Check sheet for the modelled part. Datum: model origin and axes. Units: mm. Face numbers are marked on the shaded views. A direction names the side the tool comes from. Round coordinates to 2 decimals unless told otherwise and drop trailing zeros. Order: outer loops, then holes, each group sorted by start corner. A loop starts at its lowest first (then second) coordinate and runs counter-clockwise, first axis right, second up.
(1) Mould release check, pull along X, two halves, no side actions. Record for the marked faces 4, 5, 6 and 7: released by +X, released by -X, zero draft, split by the parting line, or undercut.
(2) Sectioned sample at C-C, the plane y = 10.9. Enter the section's corners in (x, z), and give its area (3 significant figures).
(3) Thickness scan on probe 1 along X at (y, z) = (14.75, 13); probe 2 along X at (y, z) = (11, 13); probe 3 along X at (y, z) = (11.75, 13). Record the ranges inside material, lowest first.
(4) Sectioned sample at D-D, the plane z = 9.75. Enter the section's corners in (x, y).
(5) Depth check by flat-ended pin: pin 1 (1.5 mm diameter, centred on x = 20, z = 4, fed in from +Y); pin 2 (2.5 mm diameter, centred on x = 0.5, z = 13, fed in from -Y); pin 3 (3 mm diameter, centred on x = 45, z = 9.5, fed in from -Y); pin 4 (6 mm diameter, centred on x = 1.5, z = 9.5, fed in from -Y). Enter the tip coordinate at first touch or a pass-through.
(6) Sectioned sample at A-A, the plane z = 3. Enter the section's corners in (x, y).
(7) Sectioned sample at B-B, the plane x = 0.5. Enter the section's corners in (y, z), and give its area (3 significant figures).
(8) Tool access check on the marked faces 1, 2 and 3. Record the directions out of +Z, -Z, +X, -X, +Y, -Y that give a thin tool (end or side, any length) a straight path to the whole face; none if there is none.
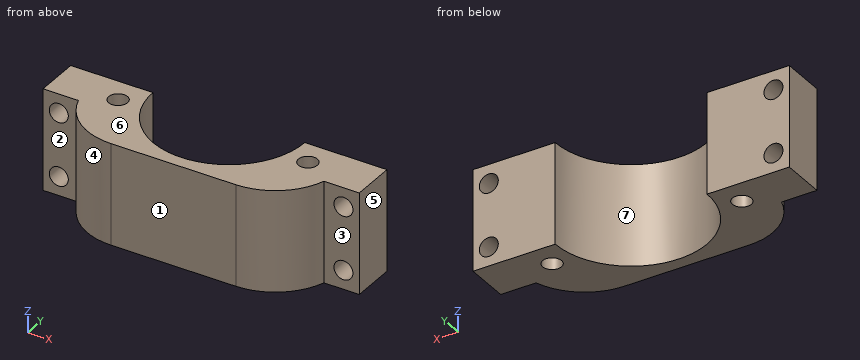
```python
from build123d import *

# Parameters (mm, degrees)
SKETCH7_R            = 1.5
BOSS_EXTRUDE11_DEPTH = 16
SKETCH8_R            = 1.5
CUT_EXTRUDE1_DEPTH   = 52.078371156
FILLET1_R            = 10


with BuildPart() as part:
    # Sketch7 → Boss-Extrude11 (new body)
    with BuildSketch(Plane.XY):
        with BuildLine():
            ThreePointArc((11, 14.9), (23, 2.9), (35, 14.9))
            Line((35, 14.9), (48, 14.9))
            Line((48, 14.9), (48, 7.9))
            Line((48, 7.9), (42.4, 7.9))
            Line((42.4, 7.9), (42.4, 0.9))
            Line((42.4, 0.9), (3.598076211, 0.9))
            Line((3.598076211, 0.9), (3.598076211, 7.9))
            Line((3.598076211, 7.9), (-2, 7.9))
            Line((-2, 7.9), (-2, 14.9))
            Line((-2, 14.9), (11, 14.9))
        make_face()
        with Locations((38, 10.9)):
            Circle(SKETCH7_R, mode=Mode.SUBTRACT)
        with Locations((8, 10.9)):
            Circle(SKETCH7_R, mode=Mode.SUBTRACT)
    extrude(amount=BOSS_EXTRUDE11_DEPTH)

    # Sketch8 → Cut-Extrude1 (cut, through all)
    with BuildSketch(Plane.XZ.offset(-7.9)):
        with Locations(Location((0.5, 13, 0), (0, 0, 270))):
            Circle(SKETCH8_R)
        with Locations(Location((45.5, 13, 0), (0, 0, 270))):
            Circle(SKETCH8_R)
        with Locations(Location((45.5, 3, 0), (0, 0, 270))):
            Circle(SKETCH8_R)
        with Locations(Location((0.5, 3, 0), (0, 0, 270))):
            Circle(SKETCH8_R)
    extrude(amount=-CUT_EXTRUDE1_DEPTH, mode=Mode.SUBTRACT)

    # Fillet1
    # the kernel refuses this fillet: 10 mm, written as the material it takes off along each edge
    with BuildSketch(Plane(origin=(3.598076211, 0.9, -23.848480035), x_dir=(1, 0, 0), z_dir=(0, 0, 1))) as fillet1_piece_1:
        with BuildLine():
            CenterArc((9.539392014, 10), FILLET1_R, 197.457603124, 72.542396876)
            Line((0, 7), (-0.19078784, 6.94))
            ThreePointArc((-0.19078784, 6.94), (-0.2, 3.5), (-0.2, 0))
            Line((-0.2, 0), (0, -0.2))
            Line((0, -0.2), (9.539392014, -0.2))
            Line((9.539392014, -0.2), (9.539392014, 0))
        make_face()
    extrude(amount=63.696960071, mode=Mode.SUBTRACT)
    with BuildSketch(Plane(origin=(42.4, 0.9, -23.848480035), x_dir=(0, 1, 0), z_dir=(0, 0, 1))) as fillet1_piece_2:
        with BuildLine():
            CenterArc((10, 9.539392014), FILLET1_R, 180, 72.542396876)
            Line((0, 9.539392014), (-0.2, 9.539392014))
            Line((-0.2, 9.539392014), (-0.2, 0))
            Line((-0.2, 0), (0, -0.2))
            ThreePointArc((0, -0.2), (3.5, -0.2), (6.94, -0.19078784))
            Line((6.94, -0.19078784), (7, 0))
        make_face()
    extrude(amount=63.696960071, mode=Mode.SUBTRACT)


solid = part.part
```
Derived:
1. face 4: released by -X
1. face 5: released by +X
1. face 6: zero draft
1. face 7: undercut
2. outline: (-2, 0) - (6.5, 0) - (6.5, 16) - (-2, 16) - close; (9.5, 0) - (11.69, 0) - (11.69, 16) - (9.5, 16) - close; (34.31, 0) - (36.5, 0) - (36.5, 16) - (34.31, 16) - close; (39.5, 0) - (48, 0) - (48, 16) - (39.5, 16) - close; hole circle Ø3 at (0.5, 3); hole circle Ø3 at (0.5, 13); hole circle Ø3 at (45.5, 3); hole circle Ø3 at (45.5, 13)
2. area: 314 mm2
3. probe 1: x = -2 to -1, 2 to 11, 35 to 44, 47 to 48
3. probe 2: x = -2 to -1, 2 to 6.5, 9.5 to 11.65, 34.35 to 36.5, 39.5 to 44, 47 to 48
3. probe 3: x = -2 to -1, 2 to 6.76, 9.24 to 11.42, 34.58 to 36.76, 39.24 to 44, 47 to 48
4. outline: (-2, 7.9) - (3.6, 7.9) arc R10 ccw to (13.14, 0.9) - (32.86, 0.9) arc R10 ccw to (42.4, 7.9) - (48, 7.9) - (48, 14.9) - (35, 14.9) arc R12 cw to (11, 14.9) - (-2, 14.9) - close; hole circle Ø3 at (8, 10.9); hole circle Ø3 at (38, 10.9)
5. pin 1: stops at y = 3.5
5. pin 2: passes through
5. pin 3: stops at y = 7.9
5. pin 4: stops at y = 5.86
6. outline: (-2, 7.9) - (-1, 7.9) - (-1, 14.9) - (-2, 14.9) - close; (2, 7.9) - (3.6, 7.9) arc R10 ccw to (13.14, 0.9) - (32.86, 0.9) arc R10 ccw to (42.4, 7.9) - (44, 7.9) - (44, 14.9) - (35, 14.9) arc R12 cw to (11, 14.9) - (2, 14.9) - close; (47, 7.9) - (48, 7.9) - (48, 14.9) - (47, 14.9) - close; hole circle Ø3 at (8, 10.9); hole circle Ø3 at (38, 10.9)
7. outline: (7.9, 0) - (14.9, 0) - (14.9, 1.5) - (7.9, 1.5) - close; (7.9, 4.5) - (14.9, 4.5) - (14.9, 11.5) - (7.9, 11.5) - close; (7.9, 14.5) - (14.9, 14.5) - (14.9, 16) - (7.9, 16) - close
7. area: 70.0 mm2
8. face 1: +Z, -Z, +X, -X, -Y
8. face 2: +Z, -Z, -X, -Y
8. face 3: +Z, -Z, +X, -Y
